Autodesk Inventor part; units mm, degrees
ref_plane "YZ Plane" through (0, 0, 0) normal (1, 0, 0) x (0, 1, 0)
ref_plane "XZ Plane" through (0, 0, 0) normal (0, 1, 0) x (-1, 0, 0)
ref_plane "XY Plane" through (0, 0, 0) normal (0, 0, 1) x (1, 0, 0)
sketch "Base" plane through (0, 0, 0) normal (0, 1, 0) x (-1, 0, 0)
  line L0 (-10.6945, 15.9529) -> (-10.6945, -124.0471)
  line L1 (5.3055, -77.3796) -> (5.3055, -30.7069)
  line L2 (-10.6945, 15.9529) -> (-5.6266, 15.9529)
  line L3 (-5.6266, 15.9529) -> (5.3055, -30.7069)
  line L4 (-10.6945, -124.0471) -> (-5.6266, -124.0471)
  line L5 (5.3055, -77.3796) -> (-5.6266, -124.0471)
  point P0 (0, 0)
  dimension "d1" = 140
extrude "Extrusion1" add sketch "Base" along normal blind 3
sketch "FrontWall" plane through (0, 3, 0) normal (0, 1, 0) x (1, 0, 0)
  line L0 (-5.3055, 30.7069) -> (5.6266, -15.9529)
  line L1 (-5.3055, 77.3796) -> (-5.3055, 30.7069)
  line L2 (5.6266, 124.0471) -> (-5.3055, 77.3796)
  line L3 (8.0997, -15.3735) -> (-2.7655, 31.0004)
  line L4 (-2.7655, 31.0004) -> (-2.7655, 77.0861)
  line L5 (-2.7655, 77.0861) -> (8.0997, 123.4677)
  line L6 (8.0997, -15.3735) -> (8.1606, -15.9529)
  line L7 (5.6266, -15.9529) -> (10.6945, -15.9529)
  line L8 (8.0997, 123.4677) -> (8.0997, 124.0471)
  line L9 (10.6945, 124.0471) -> (5.6266, 124.0471)
  point P0 (0, 0)
  dimension "d6" = 2.54
extrude "Extrusion2" add sketch "FrontWall" along normal blind 29.464
sketch "Sketch3" plane through (-5.3055, 0, -77.3796) normal (-0.9736421, 0, -0.2280812) x (-0.2280812, 0, 0.9736421)
  line L0 (-47.9308, 0) -> (-47.9308, 32.464)
  line L1 (0, 0) -> (0, 32.464)
  line L2 (-1.0536, 30.5772) -> (-46.5036, 30.5772)
  line L3 (-46.5036, 30.5772) -> (-46.5036, 10.0772)
  line L4 (-46.5036, 10.0772) -> (-1.0536, 10.0772)
  line L5 (-1.0536, 10.0772) -> (-1.0536, 30.5772)
  line L6 (-23.7786, 29.5772) -> (-28.8286, 29.5772)
  line L7 (-28.8286, 29.5772) -> (-28.8286, 25.6172)
  line L8 (-28.8286, 25.6172) -> (-18.7194, 25.6172)
  line L9 (-18.7194, 25.6172) -> (-18.7194, 29.5772)
  line L10 (-18.7194, 29.5772) -> (-23.7786, 29.5772)
  point P0 (74.13, 0)
  point P1 (-36.5036, 20.3272)
  point P2 (-11.0612, 20.3272)
  dimension "d9" = 47.9308
  dimension "d10" = 45.45
  dimension "d11" = 20.5
hole "Hole1" at (-2.7826, 20.3272, -88.1493) at (3.0203, 20.3272, -112.9211) direction (0.9736421, 0, 0.2280812) diameter 16 end through all
extrude "Extrusion3" cut sketch "Sketch3" against normal blind 29.464 contours L10 L9 L8 L7 L6
sketch "Sketch4" plane through (-5.3055, 0, -77.3796) normal (-1, 0, 0) x (0, 0, 1)
  point P0 (77.3796, 0)
sketch "Sketch5" plane through (-5.3055, 0, -77.3796) normal (-1, 0, 0) x (0, 0, 1)
  line L0 (-47.9308, 0) -> (-47.9308, 32.464)
  line L1 (0, 0) -> (0, 32.464)
  line L2 (46.1641, 30.5772) -> (0.7141, 30.5772)
  line L3 (0.7141, 30.5772) -> (0.7141, 10.0772)
  line L4 (0.7141, 10.0772) -> (46.1641, 10.0772)
  line L5 (46.1641, 10.0772) -> (46.1641, 30.5772)
  line L6 (23.4391, 29.5772) -> (18.3891, 29.5772)
  line L7 (18.3891, 29.5772) -> (18.3891, 25.6172)
  line L8 (18.3891, 25.6172) -> (28.4983, 25.6172)
  line L9 (28.4983, 25.6172) -> (28.4983, 29.5772)
  line L10 (28.4983, 29.5772) -> (23.4391, 29.5772)
  point P0 (77.3796, 0)
  point P1 (74.13, 0)
  point P2 (10.7141, 20.3272)
  point P3 (36.1565, 20.3272)
  dimension "d27" = 47.9308
  dimension "d28" = 45.45
  dimension "d29" = 20.5
hole "Hole2" at (-5.3055, 20.3272, -41.2231) at (-5.3055, 20.3272, -66.6655) direction (1, 0, 0) diameter 16 end through all
extrude "Extrusion4" cut sketch "Sketch5" against normal blind 29.464 contours L10 L9 L8 L7 L6
sketch "Sketch6" plane through (5.6266, 0, 15.9529) normal (-0.9736338, 0, 0.2281165) x (0.2281165, 0, 0.9736338)
  line L0 (-47.9308, 0) -> (-47.9308, 32.464)
  line L1 (-47.1544, 0) -> (-47.1544, 32.464)
  line L2 (-0.9903, 30.5772) -> (-46.4403, 30.5772)
  line L3 (-46.4403, 30.5772) -> (-46.4403, 10.0772)
  line L4 (-46.4403, 10.0772) -> (-0.9903, 10.0772)
  line L5 (-0.9903, 10.0772) -> (-0.9903, 30.5772)
  line L6 (-23.7153, 29.5772) -> (-28.7653, 29.5772)
  line L7 (-28.7653, 29.5772) -> (-28.7653, 25.6172)
  line L8 (-28.7653, 25.6172) -> (-18.6561, 25.6172)
  line L9 (-18.6561, 25.6172) -> (-18.6561, 29.5772)
  line L10 (-18.6561, 29.5772) -> (-23.7153, 29.5772)
  point P0 (-16.8159, 0)
  point P1 (77.3796, 0)
  point P2 (74.13, 0)
  point P3 (-36.4403, 20.3272)
  point P4 (-10.9979, 20.3272)
  dimension "d39" = 0.7874
  dimension "d40" = 45.45
  dimension "d41" = 20.5
hole "Hole3" at (-2.686, 20.3272, -19.5266) at (3.1178, 20.3272, 5.245) direction (0.9736338, 0, -0.2281165) diameter 16 end through all
extrude "Extrusion5" cut sketch "Sketch6" against normal blind 29.464 contours L10 L9 L8 L7 L6
sketch "Sketch7" plane through (0, 3, 0) normal (0, 1, 0) x (1, 0, 0)
  line L0 (10.6945, 124.0471) -> (10.6945, -15.9529)
  point P0 (0, 0)
  point P1 (2.8129, 67.1471)
  point P2 (2.8129, 40.9471)
hole "Hole4" at (2.8129, 3, -40.9471) at (2.8129, 3, -67.1471) direction (0, -1, 0) diameter 4 end through all
properties part number "UltrasonicSensorMount"
Input: part model. Units: mm. Frame: model coordinates. A direction names the side the tool comes from. Give positions to 0.01 mm unless a question says otherwise; leave off trailing zeros. Order: outer loops, then holes, each group sorted by start corner. A loop starts at its lowest first (then second) coordinate and runs counter-clockwise, first axis right, second up. Notation, with made-up numbers: (-10, 62.5) - (18, 62.5) arc R9 cw to (18, 69.5) - close; hole circle Ø9 at (-6, 68.5). An arc over 180 degrees is marked (long way). Put each result on its own line as item: value.
Item 1: Ray query, L1, parallel to Y at x = 9.5, z = -104; L2, parallel to X at y = 6, z = -77; L3, parallel to Y at x = -0.25, z = -13.5. Return the intervals inside material, ascending. Write a range as from..to.
Found:
L1: y = 0..3
L2: x = -5.31..-2.77
L3: y = 0..15.56, 25.1..32.46
Item 2: Section query C-C, the plane y = 23. Count the separate pieces of the cut face and the enclosed holes in it, then the cut area to 3 significant figures.
Found:
separate pieces: 7
enclosed holes: 0
area: 132 mm^2
Item 3: Contact query for flat-ended pins moving along their axis: pin 1 (9 mm diameter, centred on y = 20.5, z = -45.5, fed in from +X); pin 2 (12 mm diameter, centred on y = 29, z = -12.5, fed in from +X); pin 3 (3 mm diameter, centred on x = 0.5, z = -65, fed in from -Y); pin 4 (3 mm diameter, centred on x = -4, y = 26.5, fed in from +Z). Output: stop coordinate, or through.
Found:
pin 1: stops at x = -2.77
pin 2: stops at x = 2.97
pin 3: stops at y = 0
pin 4: stops at z = -22.22
Item 4: Section query D-D, the plane z = -102. Return loops of the section in (x, y).
Found:
outline: (0.46, 0) - (10.69, 0) - (10.69, 3) - (3.07, 3) - (3.07, 25.62) - (0.46, 25.62) - close; (0.46, 29.58) - (3.07, 29.58) - (3.07, 32.46) - (0.46, 32.46) - close
Item 5: Draft query along X for faces 4 (the cylindrical face through (-4, 17.9, -33.6)), 5 (the cylindrical face through (1.46, 1.48, -68.62)), 6 (the flat face through (0.18, 27.57, -95.32)). Return one class per face: +X half, -X half, draft (parallel to the pull), parting line (faces both ways), or undercut.
Found:
face 4: draft
face 5: undercut
face 6: +X half
Item 6: Access query for faces 1 (the flat face through (-4, 25.617, -54)), 2 (the flat face through (-2.766, 14, -54)), 3 (the cylindrical face through (3.976, 28.137, 3.263)). Directions: +Z, -Z, +X, -X, +Y, -Y. A direction counts if a zero-diameter tool reaches every point of the face in a straight line with its end or side. Return the directions, or none.
Found:
face 1: +X, -X
face 2: +X, +Y
face 3: none
Item 7: Section query B-B, the plane y = 9.5. Return loops of the section in (x, z), then the cut area to 3 significant figures.
Found:
outline: (-5.31, -77.38) - (5.63, -124.05) - (8.1, -124.05) - (8.1, -123.47) - (-2.77, -77.09) - (-2.77, -31) - (8.1, 15.37) - (8.16, 15.95) - (5.63, 15.95) - (-5.31, -30.71) - close
area: 362 mm^2
Item 8: Section query A-A, the plane z = -7.5. Return loops of the section in (x, y), then the cut area to 3 significant figures.
Found:
outline: (0.13, 0) - (10.69, 0) - (10.69, 3) - (2.74, 3) - (2.74, 25.62) - (0.13, 25.62) - close; (0.13, 29.58) - (2.74, 29.58) - (2.74, 32.46) - (0.13, 32.46) - close
area: 98.2 mm^2
